Here's how the part is built. I have some questions about the finished solid (model axes, mm). Face numbers are marked on the shaded views. A direction names the side the tool comes from. Coordinates: 2 decimals unless noted, no trailing zeros. Write each loop counter-clockwise with the first axis right and the second up, starting at its lowest first coordinate (ties: lowest second). Pieces come first, ordered by that corner, then holes. Notation, with made-up numbers: (13.5, -35) - (54.5, -35) arc R27 cw to (54.5, 4) - close; hole circle Ø3 at (6, 7). An arc over 180 degrees is marked (long way). Answer in a Markdown table with one row per item. Add a question column.
Item 1: We'd pull the mould along Z, two halves only. Please class the marked faces 4, 5 and 6: +Z half, -Z half, draft (parallel to the pull), parting line (faces both ways), or undercut.
Item 2: Imagine slicing it at A-A (z = -89). Please give me the cut outline in (x, y).
Item 3: I'm going to push flat-ended pins straight in: pin 1 (3 mm diameter, centred on x = -21, y = 5, fed in from +Z); pin 2 (12 mm diameter, centred on x = -86, z = -172.5, fed in from +Y); pin 3 (1.8 mm diameter, centred on x = -197, z = -3, fed in from -Y); pin 4 (5 mm diameter, centred on x = -109, y = 6, fed in from +Z). Where does each tip first touch, or does it pass through?
Item 4: Imagine slicing it at B-B (x = -116). Please give me the cut outline in (y, z), plus the area to 3 significant figures.
Item 5: Which directions (+Z, -Z, +X, -X, +Y, -Y) give clear straight access to the entire face, cutting with the end or side of a thin tool? Please do the marked faces 1, 2 and 3.
Item 6: Imagine slicing it at D-D (x = -45). Please give me the cut outline in (y, z).
Item 7: Imagine slicing it at C-C (y = 33.5). Please give me the cut outline in (x, z).
Item 8: If I drill on probe 1 along X at (y, z) = (52.35, -197); probe 2 along Z at (x, y) = (-135.5, 45), over which ranges is the centre line in solid material (lowest first)? Write a range as from..to.
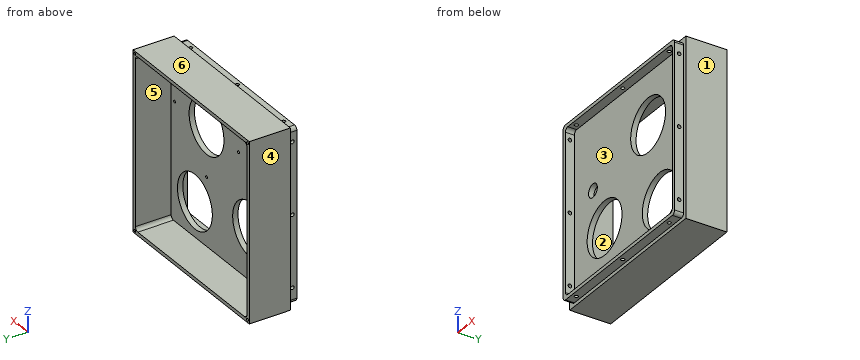
Autodesk Inventor part; units mm, degrees
ref_plane "YZ Plane" through (0, 0, 0) normal (1, 0, 0) x (0, 1, 0)
ref_plane "XZ Plane" through (0, 0, 0) normal (0, 1, 0) x (-1, 0, 0)
ref_plane "XY Plane" through (0, 0, 0) normal (0, 0, 1) x (1, 0, 0)
sketch "Sketch1" plane through (0, 0, 0) normal (0, 1, 0) x (-1, 0, 0)
  line L0 (0, 0) -> (200, 0)
  line L1 (200, 0) -> (200, -200)
  line L2 (200, -200) -> (0, -200)
  line L3 (0, -200) -> (0, 0)
  dimension "d0" = 200
  dimension "d1" = 200
extrude "Extrusion1" add sketch "Sketch1" along normal blind 56
sketch "Sketch2" plane through (0, 56, 0) normal (0, 1, 0) x (1, 0, 0)
  line L0 (-4, 4) -> (-196, 4)
  line L1 (-196, 4) -> (-196, 196)
  line L2 (-196, 196) -> (-4, 196)
  line L3 (-4, 196) -> (-4, 4)
  line L4 (0, 0) -> (0, 200)
  line L5 (-200, 0) -> (0, 0)
  dimension "d4" = 192
  dimension "d5" = 192
  dimension "d6" = 4
  dimension "d7" = 4
extrude "Extrusion2" cut sketch "Sketch2" against normal blind 40
sketch "Sketch3" plane through (0, 0, 0) normal (0, -1, 0) x (1, 0, 0)
  line L0 (-196, -4) -> (-4, -4)
  line L1 (-4, -4) -> (-4, -196)
  line L2 (-4, -196) -> (-196, -196)
  line L3 (-196, -196) -> (-196, -4)
  line L4 (-200, 0) -> (-200, -200)
  line L5 (0, 0) -> (-200, 0)
  line L6 (0, 0) -> (-200, 0)
  line L7 (-200, 0) -> (-200, -200)
  line L8 (-200, -200) -> (0, -200)
  line L9 (0, -200) -> (0, 0)
  line L10 (-8, -8) -> (-192, -8)
  line L11 (-192, -8) -> (-192, -192)
  line L12 (-192, -192) -> (-8, -192)
  line L13 (-8, -192) -> (-8, -8)
  dimension "d10" = 192
  dimension "d11" = 192
  dimension "d12" = 4
  dimension "d13" = 4
  dimension "d16" = 4
extrude "Extrusion3" cut sketch "Sketch3" against normal blind 10
fillet "Fillet1" radius 4 12 edges at (-196, 36, -196) (-196, 36, -4) (-4, 36, -196) (-4, 36, -4) (-4, 5, -4) (-4, 5, -196) (-196, 5, -196) (-196, 5, -4) (-8, 5, -192) (-8, 5, -8) (-192, 5, -192) (-192, 5, -8)
sketch "Sketch8" plane through (0, 16, 0) normal (0, 1, 0) x (1, 0, 0)
  circle A0 centre (-65, 65) radius 40
  line L0 (0, 0) -> (0, 200)
  line L1 (-200, 0) -> (0, 0)
  circle A1 centre (-140, 140) radius 37.5
  line L2 (0, 200) -> (-200, 200)
  line L3 (-200, 200) -> (-200, 0)
  circle A2 centre (-140, 140) radius 55
  line L4 (-185, 78) -> (-135, 78)
  line L5 (-135, 78) -> (-135, 10)
  line L6 (-135, 10) -> (-185, 10)
  line L7 (-185, 10) -> (-185, 78)
  circle A3 centre (-65, 65) radius 50
  circle A4 centre (-65, 65) radius 60
  line L8 (-185, 19) -> (-135, 19)
  line L9 (-135, 19) -> (-135, 69)
  line L10 (-135, 69) -> (-185, 69)
  line L11 (-185, 69) -> (-185, 19)
  circle A5 centre (-140, 140) radius 30
  circle A6 centre (-45, 157) radius 30
  circle A7 centre (-65, 65) radius 30
  circle A8 centre (-160, 89) radius 7.5
  line L12 (0, 0) -> (0, 200)
  line L13 (-200, 0) -> (0, 0)
  dimension "d152" = 80
  dimension "d153" = 65
  dimension "d154" = 65
  dimension "d155" = 75
  dimension "d156" = 140
  dimension "d157" = 140
  dimension "d158" = 110
  dimension "d159" = 50
  dimension "d160" = 68
  dimension "d161" = 10
  dimension "d162" = 100
  dimension "d163" = 120
  dimension "d164" = 135
  dimension "d165" = 50
  dimension "d166" = 50
  dimension "d167" = 9
  dimension "d168" = 60
  dimension "d169" = 60
  dimension "d170" = 60
  dimension "d171" = 15
  dimension "d172" = 20
  dimension "d173" = 25
  dimension "d174" = 45
  dimension "d175" = 157
extrude "Extrusion4" cut sketch "Sketch8" against normal through all contours A8 A2 | A2 A8 | A5 | A6 | A7
sketch "Sketch4" plane through (0, 56, 0) normal (0, 1, 0) x (1, 0, 0)
  circle A0 centre (-197, 197) radius 1.5
  line L0 (0, 200) -> (-200, 200)
  line L1 (-200, 200) -> (-200, 0)
  circle A1 centre (-197, 3) radius 1.5
  line L2 (-200, 0) -> (0, 0)
  circle A2 centre (-3, 197) radius 1.5
  line L3 (0, 0) -> (0, 200)
  circle A3 centre (-3, 3) radius 1.5
  dimension "d18" = 3
  dimension "d19" = 3
  dimension "d20" = 3
  dimension "d21" = 3
  dimension "d22" = 3
  dimension "d23" = 3
  dimension "d24" = 3
  dimension "d25" = 3
  dimension "d26" = 3
  dimension "d27" = 3
  dimension "d28" = 3
  dimension "d29" = 3
hole "Hole1" at (-197, 56, -3) at (-197, 56, -197) at (-3, 56, -197) at (-3, 56, -3) direction (0, -1, 0) diameter 3 depth 5 tip angle 118
sketch "Sketch5" plane through (-4, 0, -8) normal (1, 0, 0) x (0, 0, -1)
  circle A0 centre (11, 5) radius 2
  line L0 (184, 0) -> (0, 0)
  circle A1 centre (91, 5) radius 2
  circle A2 centre (171, 5) radius 2
  line L1 (-4, 10) -> (-4, 0)
  line L2 (-4, 0) -> (-4, 10)
  line L3 (-4, 10) -> (-4, 0)
  line L4 (0, 0) -> (0, 10)
  dimension "d37" = 4
  dimension "d38" = 5
  dimension "d42" = 80
  dimension "d54" = 11
hole "Hole2" at (-4, 5, -19) at (-4, 5, -99) at (-4, 5, -179) direction (-1, 0, 0) diameter 4 end through all
sketch "Sketch6" plane through (-192, 0, -4) normal (0, 0, 1) x (1, 0, 0)
  circle A0 centre (11, 5) radius 2
  line L0 (182, 0) -> (0, 0)
  line L1 (-4, 0) -> (-4, 10)
  circle A1 centre (91, 5) radius 2
  circle A2 centre (171, 5) radius 2
  line L2 (-4, 10) -> (-4, 0)
  line L3 (-4, 0) -> (-4, 10)
  line L4 (-4, 10) -> (-4, 0)
  line L5 (0, 0) -> (0, 10)
  point P0 (192, 0)
  point P1 (186, 0)
  dimension "d59" = 4
  dimension "d60" = 5
  dimension "d61" = 80
  dimension "d62" = 11
hole "Hole3" at (-181, 5, -4) at (-101, 5, -4) at (-21, 5, -4) direction (0, 0, -1) diameter 4 end through all
sketch "Sketch7" plane through (0, 16, 0) normal (0, 1, 0) x (1, 0, 0)
  line L0 (-200, 200) -> (-200, 0)
  line L1 (-200, 0) -> (0, 0)
  line L2 (-185, 78) -> (-135, 78)
  line L3 (-135, 78) -> (-135, 10)
  line L4 (-135, 10) -> (-185, 10)
  line L5 (-185, 10) -> (-185, 78)
  line L6 (0, 0) -> (0, 200)
  line L7 (-185, 78) -> (-173, 78)
  line L8 (-173, 78) -> (-173, 10)
  line L9 (-173, 10) -> (-185, 10)
  line L10 (-185, 10) -> (-185, 78)
  line L11 (-135, 78) -> (-147, 78)
  line L12 (-147, 78) -> (-147, 10)
  line L13 (-147, 10) -> (-135, 10)
  line L14 (-135, 10) -> (-135, 78)
  circle A0 centre (-179, 63) radius 2
  circle A1 centre (-179, 25) radius 2
  circle A2 centre (-141, 63) radius 2
  circle A3 centre (-141, 25) radius 2
  circle A4 centre (-65, 65) radius 60
  circle A5 centre (-65, 65) radius 55
  circle A6 centre (-65, 120) radius 2
  circle A7 centre (-120, 65) radius 2
  circle A8 centre (-65, 10) radius 2
  circle A9 centre (-10, 65) radius 2
  dimension "d106" = 110
  dimension "d74" = 50
  dimension "d75" = 68
  dimension "d76" = 10
  dimension "d79" = 135
  dimension "d80" = 12
  dimension "d81" = 68
  dimension "d82" = 12
  dimension "d83" = 68
  dimension "d84" = 4
  dimension "d85" = 4
  dimension "d86" = 4
  dimension "d87" = 4
  dimension "d88" = 15
  dimension "d89" = 15
  dimension "d90" = 15
  dimension "d91" = 15
  dimension "d92" = 6
  dimension "d93" = 6
  dimension "d94" = 6
  dimension "d95" = 6
  dimension "d103" = 120
  dimension "d104" = 65
  dimension "d105" = 65
  dimension "d107" = 4
  dimension "d110" = 360
hole "Hole4" at (-179, 16, -63) at (-141, 16, -63) at (-179, 16, -25) at (-141, 16, -25) at (-65, 16, -120) at (-120, 16, -65) at (-65, 16, -10) at (-10, 16, -65) direction (0, -1, 0) diameter 3 depth 5 tip angle 118
thread "Thread1"
thread "Thread2"
thread "Thread3"
thread "Thread4"
thread "Thread5"
thread "Thread6"
thread "Thread7"
thread "Thread8"
thread "Thread9"
thread "Thread10"
thread "Thread11"
thread "Thread12"
thread "Thread13"
thread "Thread14"
thread "Thread15"
thread "Thread16"
thread "Thread17"
thread "Thread18"
thread "Thread19"
thread "Thread20"
thread "Thread21"
thread "Thread22"
thread "Thread23"
thread "Thread24"
properties part number "Housing_top" material "Aluminum 6061"
Here are the results:
| question | item | result |
|---|---|---|
| 1 | face 4 | draft |
| 1 | face 5 | undercut |
| 1 | face 6 | +Z half |
| 2 | outline | (-200, 10) - (-196, 10) - (-196, 0) - (-192, 0) - (-192, 10) - (-167.5, 10) - (-167.5, 16) - (-196, 16) - (-196, 56) - (-200, 56) - close; (-152.5, 10) - (-83, 10) - (-83, 16) - (-152.5, 16) - close; (-47, 10) - (-8, 10) - (-8, 0) - (-4, 0) - (-4, 10) - (0, 10) - (0, 56) - (-4, 56) - (-4, 16) - (-47, 16) - close |
| 3 | pin 1 | passes through |
| 3 | pin 2 | stops at y = 16 |
| 3 | pin 3 | stops at y = 10 |
| 3 | pin 4 | stops at z = -4 |
| 4 | outline | (0, -196) - (10, -196) - (10, -200) - (56, -200) - (56, -196) - (16, -196) - (16, -158) - (10, -158) - (10, -192) - (0, -192) - close; (0, -8) - (10, -8) - (10, -122) - (16, -122) - (16, -4) - (56, -4) - (56, 0) - (10, 0) - (10, -4) - (0, -4) - close |
| 4 | area | 1,380 mm2 |
| 5 | face 1 | +Z, -Z, +X, +Y, -Y |
| 5 | face 2 | +Y |
| 5 | face 3 | -Y |
| 6 | outline | (0, -196) - (10, -196) - (10, -200) - (56, -200) - (56, -196) - (16, -196) - (16, -187) - (10, -187) - (10, -192) - (0, -192) - close; (0, -8) - (10, -8) - (10, -42.64) - (16, -42.64) - (16, -4) - (56, -4) - (56, 0) - (10, 0) - (10, -4) - (0, -4) - close; (10, -127) - (16, -127) - (16, -87.36) - (10, -87.36) - close |
| 7 | outline | (-200, -200) - (0, -200) - (0, 0) - (-200, 0) - close; hole (-196, -192) arc R4 ccw to (-192, -196) - (-8, -196) arc R4 ccw to (-4, -192) - (-4, -8) arc R4 ccw to (-8, -4) - (-192, -4) arc R4 ccw to (-196, -8) - close |
| 8 | probe 1 | x = -200..-198.5, -195.5..-4.5, -1.5..0 |
| 8 | probe 2 | z = -200..-196, -4..0 |
